from build123d import *

# Parameters (mm, degrees)
F0_W     = 484
F0_H     = 325
F1_DEPTH = 6
F3_D     = 12.5


with BuildPart() as f1:
    # F0 (on Front) → F1 (new body)
    with BuildSketch(Plane.XZ):
        with BuildLine():
            Line((-287, -217.5), (287, -217.5))
            ThreePointArc((287, -217.5), (290.5355339059, -216.0355339059), (292, -212.5))
            Line((292, -212.5), (292, 212.5))
            ThreePointArc((292, 212.5), (290.5355339059, 216.0355339059), (287, 217.5))
            Line((287, 217.5), (-287, 217.5))
            ThreePointArc((-287, 217.5), (-290.5355339059, 216.0355339059), (-292, 212.5))
            Line((-292, 212.5), (-292, -212.5))
            ThreePointArc((-292, -212.5), (-290.5355339059, -216.0355339059), (-287, -217.5))
        make_face()
        Rectangle(F0_W, F0_H, mode=Mode.SUBTRACT)
    extrude(amount=F1_DEPTH)

    # F3 (through all)
    with Locations(Plane(origin=(0, 0, 0), x_dir=(1, 0, 0), z_dir=(0, 1, 0))):
        with Locations((-272, -192.45), (-272, -64.15), (-272, 64.15), (-272, 192.45), (-136, 192.45), (0, 192.45), (272, 192.45), (136, 192.45), (272, -64.15), (272, 64.15), (272, -192.45), (-136, -192.45), (136, -192.45), (0, -192.45)):
            Hole(F3_D / 2)


solid = f1.part
Geometry: final body of the model. Coordinates: model frame, mm. Give positions to 0.01 mm unless a question says otherwise; leave off trailing zeros. Write each loop counter-clockwise with the first axis right and the second up, starting at its lowest first coordinate (ties: lowest second). Pieces come first, ordered by that corner, then holes.
(1) Cut plane B-B, the plane x = 272. Return loops of the section in (y, z), then the cut area to 3 significant figures.
(2) Cut plane D-D, the plane x = 136. Return loops of the section in (y, z), then the cut area to 3 significant figures.
(3) Cut plane A-A, the plane z = -64.15. Return loops of the section in (x, y).
(4) Mould query, pull axis Z, two halves, no side actions, for faces 1 (the cylindrical face through (276.96, -3.04, 196.25)), 2 (the flat face through (-1, -6, -176)). Classes: released by +Z, released by -Z, zero draft, split by the parting line, or undercut.
(5) Cut plane C-C, the plane z = -1.5. Return loops of the section in (x, y).
(6) Ray query, line 1 (Z direction, x = 136, y = -4.45); line 2 (X direction, y = -4.7, z = 64.15); line 3 (Z direction, x = 272, y = -4.1). Return the intervals inside material, ascending.
Values follow:
1. outline: (-6, -217.5) - (0, -217.5) - (0, -198.7) - (-6, -198.7) - close; (-6, -186.2) - (0, -186.2) - (0, -70.4) - (-6, -70.4) - close; (-6, -57.9) - (0, -57.9) - (0, 57.9) - (-6, 57.9) - close; (-6, 70.4) - (0, 70.4) - (0, 186.2) - (-6, 186.2) - close; (-6, 198.7) - (0, 198.7) - (0, 217.5) - (-6, 217.5) - close
1. area: 2,310 mm2
2. outline: (-6, -217.5) - (0, -217.5) - (0, -198.7) - (-6, -198.7) - close; (-6, -186.2) - (0, -186.2) - (0, -162.5) - (-6, -162.5) - close; (-6, 162.5) - (0, 162.5) - (0, 186.2) - (-6, 186.2) - close; (-6, 198.7) - (0, 198.7) - (0, 217.5) - (-6, 217.5) - close
2. area: 510 mm2
3. outline: (-292, -6) - (-278.25, -6) - (-278.25, 0) - (-292, 0) - close; (-265.75, -6) - (-242, -6) - (-242, 0) - (-265.75, 0) - close; (242, -6) - (265.75, -6) - (265.75, 0) - (242, 0) - close; (278.25, -6) - (292, -6) - (292, 0) - (278.25, 0) - close
4. face 1: undercut
4. face 2: zero draft
5. outline: (-292, -6) - (-242, -6) - (-242, 0) - (-292, 0) - close; (242, -6) - (292, -6) - (292, 0) - (242, 0) - close
6. line 1: z = -217.5 to -198.7, -186.2 to -162.5, 162.5 to 186.2, 198.7 to 217.5
6. line 2: x = -292 to -278.25, -265.75 to -242, 242 to 265.75, 278.25 to 292
6. line 3: z = -217.5 to -198.7, -186.2 to -70.4, -57.9 to 57.9, 70.4 to 186.2, 198.7 to 217.5
